Part print with two shaded views. Sizes in mm from the minimum x, y, z corner. A direction names the side the tool comes from. Give positions to 0.01 mm unless a question says otherwise; leave off trailing zeros. Order: outer loops, then holes, each group sorted by start corner. A loop starts at its lowest first (then second) coordinate and runs counter-clockwise, first axis right, second up. Notation, with made-up numbers: (68.25, -17.75) -> (77.25, -17.75) arc R35 ccw to (77.25, 18.25) -> close; hole circle Ø10 at (-24.75, -21.5). An arc over 180 degrees is marked (long way). Answer as CSV lines item,"result".
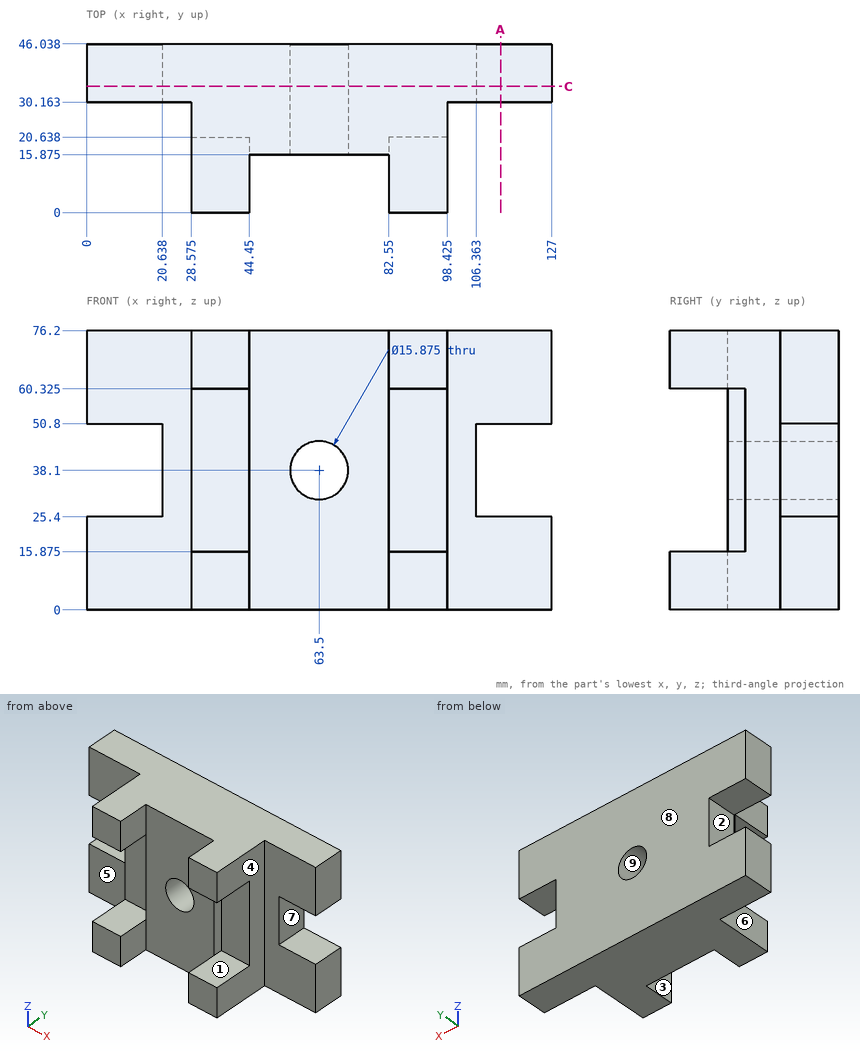
1) Which spindle directions (+Z, -Z, +X, -X, +Y, -Y) get a long thin tool onto all of the face, cutting with end or side? Do the marked faces 1, 2, 3, 4 and 5. Say none if no direction does.
Data:
face 1,"+X, -Y"
face 2,"-X, +Y, -Y"
face 3,"+Z, -Z, -Y"
face 4,"+Z, -Z, +X, -Y"
face 5,"+Z, -Z, -X, -Y"
2) Band-saw the part on A-A, the plane x = 113. Write the cut outline in (y, z).
Data:
outline,"(30.16, 0) -> (46.04, 0) -> (46.04, 25.4) -> (30.16, 25.4) -> close; (30.16, 50.8) -> (46.04, 50.8) -> (46.04, 76.2) -> (30.16, 76.2) -> close"
3) Wall check: line 1 along Z through (x, y) = (63.5, 30); line 2 along X through (y, z) = (30, 38) (1 decimal); line 3 along Y through (x, z) = (62.5, 59.5) (1 decimal). Give the ranges that are in metal, low to high. Write a range as [from, to].
Data:
line 1,"z = [0, 30.16], [46.04, 76.2]"
line 2,"x = [28.6, 55.6], [71.4, 98.4]"
line 3,"y = [15.9, 46]"
4) Pull direction X, two halves, no side cores. Call the marked faces 6, 7, 8 and 9: pulls with the +X half, pulls with the -X half, needs draft (parallel to the pull), parting line crosses it, or undercut.
Data:
face 6,"pulls with the -X half"
face 7,"pulls with the +X half"
face 8,"needs draft"
face 9,"undercut"
5) Band-saw the part on C-C, the plane y = 34.5. Write the cut outline in (x, z) (1 decimal), then the cut area to 3 significant figures.
Data:
outline,"(0, 0) -> (127, 0) -> (127, 25.4) -> (106.4, 25.4) -> (106.4, 50.8) -> (127, 50.8) -> (127, 76.2) -> (0, 76.2) -> (0, 50.8) -> (20.6, 50.8) -> (20.6, 25.4) -> (0, 25.4) -> close; hole circle Ø15.9 at (63.5, 38.1)"
area,"8,430 mm2"
6) Pin check, flat tips, straight feed: P1, Ø14.5, axis at x = 63.5, z = 38.1, coming from the +Y side; P2, Ø5, axis at y = 18.5, z = 43.5, coming from the -X side (1 decimal); P3, Ø23, axis at x = 9, z = 25.5, coming from the -Y side; P4, Ø10, axis at x = 88, y = 22, coming from the -Z side. Stop position of each tip, or through.
Data:
P1,"passes through"
P2,"stops at x = 28.6"
P3,"stops at y = 30.16"
P4,"stops at z = 0"
